Could you check a few things on this model? Use its own coordinates, in mm. A direction names the side the tool comes from. Give positions to 0.01 mm unless a question says otherwise; leave off trailing zeros. Order: outer loops, then holes, each group sorted by start corner. A loop starts at its lowest first (then second) coordinate and runs counter-clockwise, first axis right, second up. Notation, with made-up numbers: M 68.25,70.5 L 92.25,70.5 A18 cw 92.25,90.5 Z; hole C -10,7.25 d2. An arc over 180 degrees is marked long. Answer in a Markdown table with one row per item. Add a question column.
```python
from build123d import *

# Parameters (mm, degrees)
SKETCH8_R           = 12.445803737
BOSS_EXTRUDE2_DEPTH = 7.961436264
SKETCH10_R          = 2.110408374
CUT_EXTRUDE1_DEPTH  = 137.414


with BuildPart() as part:
    # Sketch3 → Revolve2 (revolve)
    with BuildSketch(Plane(origin=(0, 0, 0), x_dir=(0, 0, -1), z_dir=(1, 0, 0)), mode=Mode.PRIVATE) as revolve2_sk:
        Polygon((29.100336298, 44.026196045), (-29.100336298, 44.026196045), (-30.085520968, 52.11445688), (-36.460084033, 52.11445688), (-35.478243613, 40.988977361), (35.478243613, 40.988977361), (36.460084033, 52.11445688), (30.085520968, 52.11445688), align=None)
    revolve(revolve2_sk.sketch.rotate(Axis((0, 4.491617138, 34.868994977), (0, 0, -1)), 90), axis=Axis((0, 4.491617138, 34.868994977), (0, 0, -1)))



with BuildPart() as body_2:
    # Sketch8 → Boss-Extrude2 (new body)
    with BuildSketch(Plane.XY.offset(22.147154131)):
        with Locations((0, 4.491617138)):
            Circle(SKETCH8_R)
    extrude(amount=BOSS_EXTRUDE2_DEPTH)

    # Sketch10 → Cut-Extrude1 (cut)
    with BuildSketch(Plane.XY.offset(40.64)):
        with Locations((0, 13.095758201)):
            Circle(SKETCH10_R)
        with Locations((7.407159638, 7.714141713)):
            Circle(SKETCH10_R)
        with Locations((4.577876416, -0.99349668)):
            Circle(SKETCH10_R)
        with Locations((-4.577876416, -0.99349668)):
            Circle(SKETCH10_R)
        with Locations((-7.407159638, 7.714141713)):
            Circle(SKETCH10_R)
    extrude(amount=-CUT_EXTRUDE1_DEPTH, mode=Mode.SUBTRACT)


with BuildPart() as part_1:
    add(part.part)

    add(body_2.part)  # Revolve4 merges body 2
    # Sketch12 → Revolve4 (revolve)
    with BuildSketch(Plane(origin=(0, 0, 0), x_dir=(0, 0, -1), z_dir=(1, 0, 0)), mode=Mode.PRIVATE) as revolve4_sk:
        with BuildLine():
            Line((-29.100336298, 42.19314735), (-26.54142097, 42.19314735))
            add(Edge.make_bspline(
                [(-26.54142097, 42.19314735), (-29.106417972, 28.876495724), (-26.54142097, 15.583923694)],
                knots=[0, 0, 0, 1, 1, 1], degree=2))
            Line((-26.54142097, 15.583923694), (-29.100336298, 15.583923694))
            add(Edge.make_bspline(
                [(-29.100336298, 42.19314735), (-31.192110403, 28.880503774), (-29.100336298, 15.583923694)],
                knots=[0, 0, 0, 1, 1, 1], degree=2))
        make_face()
    revolve(revolve4_sk.sketch.rotate(Axis((0, 4.491617138, 34.868994977), (0, 0, -1)), 90), axis=Axis((0, 4.491617138, 34.868994977), (0, 0, -1)))


solid = part_1.part
```
1. Will these pins go through, and if not, where does the flat tip stop? P1, Ø6, axis at x = -24, y = 11.5, coming from the -Z side; P2, Ø7, axis at x = 0, y = 13.1, coming from the -Z side; P3, Ø1.5, axis at y = -32.5, z = -2.5, coming from the -X side.
2. Suppose I cut it at A-A on z = -27. List the corners of the cut face in (x, y) for me, plus the area to 3 significant figures.
3. Thinking about a two-plate mould opening in Z: for faces 1 (the cylindrical face through (-47.577, 2.398, -33.228)), 2 (the cylindrical face through (-31.37, 28.55, 0.41)), 3 (the flat face through (0, 5, 30.109)), which applies, pulls with the +Z half, pulls with the -Z half, needs draft (parallel to the pull), parting line crosses it, or undercut?
4. If I drill on line 1 along Y through (x, z) = (0, 25.25); line 2 along X through (y, z) = (15, 24.5); line 3 along Z through (x, y) = (4, 14.5), over which ranges is the centre line in solid material (lowest first)? Write a range as [from, to].
5. For faces 4 (the cylindrical face through (-4.751, -31.695, 32.336)), 5 (the cylindrical face through (3.02, 0.43, 26.18)), 6 (the conical face through (-8.68, 43.58, 29.16)), 7 (the cylindrical face through (-2.698, -7.658, 24.436)), which set-ups out of +Z, -Z, +X, -X, +Y, -Y let a thin tool reach every point of the face, with its end or its side?
Findings below:
| question | item | result |
|---|---|---|
| 1 | P1 | z = 27.73 |
| 1 | P2 | z = 22.15 |
| 1 | P3 | x = -15.8 |
| 2 | outline | C 0,4.49 d79.07; hole C 0,4.49 d72.99 |
| 2 | area | 725 mm2 |
| 3 | face 1 | needs draft |
| 3 | face 2 | undercut |
| 3 | face 3 | pulls with the +Z half |
| 4 | line 1 | [-35.04, -32.01], [-7.95, 10.99], [15.21, 16.94], [40.99, 44.03] |
| 4 | line 2 | [-38.11, -34.95], [-6.67, -0.91], [0.91, 6.67], [34.95, 38.11] |
| 4 | line 3 | [22.15, 30.11] |
| 5 | face 4 | +Z |
| 5 | face 5 | +Z, -Z |
| 5 | face 6 | none |
| 5 | face 7 | -Z |
